```python
from build123d import *

# Parameters (mm, degrees)
F0_W     = 101.6
F0_H     = 76.2
F1_DEPTH = 12.7
F2_W     = 95.25
F2_H     = 69.85
F3_DEPTH = 6.35
F4_W     = 76.2
F4_H     = 38.1
F5_DEPTH = 25.4


with BuildPart() as f1:
    # F0 (on Top) → F1 (new body)
    with BuildSketch(Plane.XY):
        Rectangle(F0_W, F0_H)
    extrude(amount=F1_DEPTH)

    # F2 (on face) → F3 (cut)
    with BuildSketch(Plane(origin=(0, 0, 0), x_dir=(1, 0, 0), z_dir=(0, 0, -1))):
        with Locations((3.175, -3.175)):
            Rectangle(F2_W, F2_H)
    extrude(amount=-F3_DEPTH, mode=Mode.SUBTRACT)

    # F4 (on face) → F5 (cut)
    with BuildSketch(Plane.XY.offset(12.7)):
        with Locations((6.35, 0)):
            Rectangle(F4_W, F4_H)
    extrude(amount=-F5_DEPTH, mode=Mode.SUBTRACT)


solid = f1.part
```
Input: part model. Units: mm. Frame: model coordinates. A direction names the side the tool comes from. Coordinates: 2 decimals unless noted, no trailing zeros. Loops run counter-clockwise (first coordinate to the right, second up) from the corner with the lowest first, then second, coordinate; pieces in that order, holes last. Notation, with made-up numbers: M 58,55 L 84,55 A14 cw 84,63 Z; hole C -1,85 d9. An arc over 180 degrees is marked long. Use a Markdown table: item, result. Add a question column.
1) Pin query (flat end, axial travel): P1, Ø3, axis at x = 2, z = 4.5, coming from the +Y side; P2, Ø2, axis at y = -16.5, z = 2, coming from the +X side. Return the tip coordinate at first contact, or that it passes through.
2) Section C-C, the plane z = 11. Return the cut outline in (x, y).
3) Section D-D, the plane z = 1.75. Return the cut outline in (x, y), plus the area to 3 significant figures.
4) Line query: L1, parallel to Y at x = 12, z = 9; L2, parallel to X at y = -15, z = 8.75; L3, parallel to X at y = -26, z = 1.25. Output: solid intervals per line, ascending. Write a range as from..to.
5) Set-up query: faces 5 (the flat face through (3, -31.75, 3)), 6 (the flat face through (-31.75, 0, 10)), 7 (the flat face through (-35, 1, 12.7)). Return all of +Z, -Z, +X, -X, +Y, -Y with unobstructed straight access to the full face (end or side cutting, diameter ignored); none if empty.
6) Section B-B, the plane x = 10. Return the cut outline in (y, z), plus the area to 3 significant figures.
7) Section A-A, the plane y = -15.5. Return the cut outline in (x, z), plus the area to 3 significant figures.
8) Draft query along X for faces 1 (the flat face through (-44.45, 4, 3)), 2 (the flat face through (-50.8, -1, 6)), 3 (the flat face through (44.45, 0, 10)), 4 (the flat face through (3, -21, 6.35)). Return one class per face: +X half, -X half, draft (parallel to the pull), parting line (faces both ways), or undercut.
Answer below:
| question | item | result |
|---|---|---|
| 1 | P1 | y = -31.75 |
| 1 | P2 | x = -44.45 |
| 2 | outline | M -50.8,-38.1 L 50.8,-38.1 L 50.8,38.1 L -50.8,38.1 Z; hole M -31.75,-19.05 L 44.45,-19.05 L 44.45,19.05 L -31.75,19.05 Z |
| 3 | outline | M -50.8,-38.1 L 50.8,-38.1 L 50.8,-31.75 L -44.45,-31.75 L -44.45,38.1 L -50.8,38.1 Z |
| 3 | area | 1,090 mm2 |
| 4 | L1 | -38.1..-19.05, 19.05..38.1 |
| 4 | L2 | -50.8..-31.75, 44.45..50.8 |
| 4 | L3 | -50.8..-44.45 |
| 5 | face 5 | -Z, +X, +Y |
| 5 | face 6 | +Z, -Z |
| 5 | face 7 | +Z, +X, -X, +Y, -Y |
| 6 | outline | M -38.1,0 L -31.75,0 L -31.75,6.35 L -19.05,6.35 L -19.05,12.7 L -38.1,12.7 Z; M 19.05,6.35 L 38.1,6.35 L 38.1,12.7 L 19.05,12.7 Z |
| 6 | area | 282 mm2 |
| 7 | outline | M -50.8,0 L -44.45,0 L -44.45,6.35 L -31.75,6.35 L -31.75,12.7 L -50.8,12.7 Z; M 44.45,6.35 L 50.8,6.35 L 50.8,12.7 L 44.45,12.7 Z |
| 7 | area | 202 mm2 |
| 8 | face 1 | +X half |
| 8 | face 2 | -X half |
| 8 | face 3 | undercut |
| 8 | face 4 | draft |
